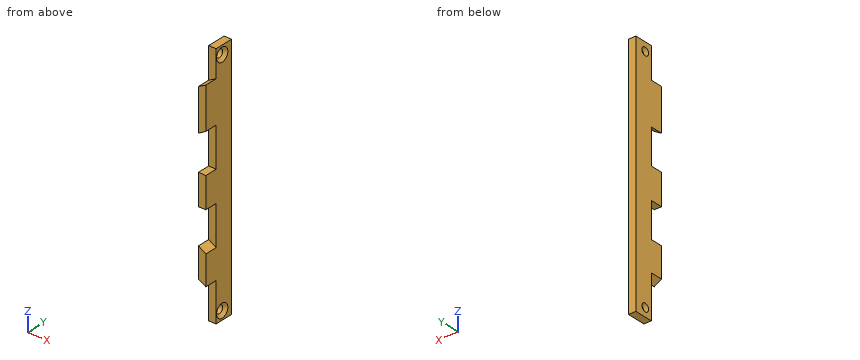
Autodesk Inventor part; units mm, degrees
ref_plane "Płaszczyzna konstrukcyjna1" through (-44.8489, 12.5303, -7) normal (0, 1, 0) x (0, 0, 1)
ref_plane "YZ Plane" through (0, 0, 0) normal (1, 0, 0) x (0, 1, 0)
ref_plane "XZ Plane" through (0, 0, 0) normal (0, 1, 0) x (-1, 0, 0)
sketch "Szkic1" plane through (0, 0, 0) normal (1, 0, 0) x (0, 1, 0)
  line L0 (0, 0) -> (10.93, 0)
  line L1 (10.93, 0) -> (10.93, -100)
  line L2 (10.93, -100) -> (0, -100)
  line L3 (0, -100) -> (0, 0)
  dimension "d0" = 10.93
  dimension "d1" = 100
extrude "Wyciągnięcie proste1" add sketch "Szkic1" along normal blind 3
sketch "Szkic2" plane through (0, 0, -100) normal (0, -1, 0) x (1, 0, 0)
  line L0 (-5, 84) -> (-8.1113, 87.1113)
  line L1 (-5, 84) -> (-4.2222, 84.7778)
  line L2 (-8.1113, 87.1113) -> (-7.3335, 87.8891)
  line L3 (-2, 60) -> (-3.1388, 64.2501)
  line L4 (-2, 60) -> (-0.9375, 60.2847)
  line L5 (-3.1388, 64.2501) -> (-2.0763, 64.5348)
  line L6 (-3.1388, 35.7499) -> (-2, 40)
  line L7 (-3.1388, 35.7499) -> (-2.0763, 35.4652)
  line L8 (-2, 40) -> (-0.9375, 39.7153)
  line L9 (-8.1113, 12.8887) -> (-5, 16)
  line L10 (-8.1113, 12.8887) -> (-7.3335, 12.1109)
  line L11 (-5, 16) -> (-4.2222, 15.2222)
  line L12 (-30.0489, 4.1) -> (-25.6489, 4.1)
  line L13 (-30.0489, 4.1) -> (-30.0489, 3)
  line L14 (-25.6489, 4.1) -> (-25.6489, 3)
  line L15 (-1.7913, 81.5519) -> (-5, 78.3431)
  line L16 (-5, 78.3431) -> (-13.7681, 87.1113)
  line L17 (-13.7681, 87.1113) -> (-10.5594, 90.32)
  line L18 (-10.5594, 90.32) -> (185.0217, 443.1577)
  arc A0 (351.0464, 277.133) -> (185.0217, 443.1577) centre (-11.203, 80.9083) ccw
  line L19 (351.0464, 277.133) -> (-1.7913, 81.5519)
  arc A1 (402.9118, 49.2349) -> (342.1425, 276.0288) centre (-8.9178, 60.424) ccw
  line L20 (402.9118, 49.2349) -> (-0.4452, 56.2755)
  line L21 (-0.4452, 56.2755) -> (-4.8284, 55.101)
  line L22 (-4.8284, 55.101) -> (-8.0378, 67.0785)
  line L23 (-8.0378, 67.0785) -> (-3.6546, 68.253)
  line L24 (-3.6546, 68.253) -> (342.1425, 276.0288)
  arc A2 (342.1425, -176.0288) -> (402.9118, 50.7651) centre (-8.9178, 39.576) ccw
  line L25 (342.1425, -176.0288) -> (-3.6546, 31.747)
  line L26 (-3.6546, 31.747) -> (-8.0378, 32.9215)
  line L27 (-8.0378, 32.9215) -> (-4.8284, 44.899)
  line L28 (-4.8284, 44.899) -> (-0.4452, 43.7245)
  line L29 (-0.4452, 43.7245) -> (402.9118, 50.7651)
  arc A3 (185.0217, -343.1577) -> (351.0464, -177.133) centre (-11.203, 19.0917) ccw
  line L30 (185.0217, -343.1577) -> (-10.5594, 9.68)
  line L31 (-10.5594, 9.68) -> (-13.7681, 12.8887)
  line L32 (-13.7681, 12.8887) -> (-5, 21.6569)
  line L33 (-5, 21.6569) -> (-1.7913, 18.4481)
  line L34 (-1.7913, 18.4481) -> (351.0464, -177.133)
  line L35 (-25.6489, 3) -> (-30.0489, 3)
  line L36 (-0.9375, 39.7153) -> (-2.0763, 35.4652)
  line L37 (-7.3335, 87.8891) -> (-4.2222, 84.7778)
  line L38 (-4.2222, 15.2222) -> (-7.3335, 12.1109)
  line L39 (-2.0763, 64.5348) -> (-0.9375, 60.2847)
  point P0 (0, 100)
  point P1 (259.8393, 226.5761)
  point P2 (359.0779, 50)
  point P3 (259.8393, -126.5761)
  point P4 (343.886, -173.1639)
  point P5 (402.9318, 50)
  point P6 (343.886, 273.1639)
extrude "Wyciągnięcie proste2" cut sketch "Szkic2" against normal blind 5 contours L0 L2 L37 L1 | L3 L5 L39 L4 | L6 L8 L36 L7 | L9 L11 L38 L10 | L15 L16 L17 L18 A0 L19 A1 L24 | L24 A1 L19 | L19 A1 A2 L29 L20 L21 L22 L23 L24 | A2 L34 L25 L26 L27 L28 L29 L20 A1 | A1 L20 L29 A2 | L34 A3 L30 L31 L32 L33 L25 A2 | A2 L25 L34
sketch "Szkic3" plane through (3, 0, 0) normal (1, 0, 0) x (0, 0, -1)
  circle A0 centre (3.5, 7.9652) radius 2
  circle A1 centre (96.5, 7.9652) radius 2
  point P0 (0, 0)
hole "Otwór1" at (3, 7.9652, -3.5) at (3, 7.9652, -96.5) direction (-1, 0, 0) diameter 3.2 depth 5 tip angle 118 countersink diameter 5.5 countersink angle 90
sketch "Szkic4" plane through (0, 5, -100) normal (0, -1, 0) x (1, 0, 0)
  line L0 (3, 100) -> (3, 84.2077)
  line L1 (0, 100) -> (3, 100)
  line L2 (0, 82.5448) -> (0, 100)
  line L3 (3, 84.2077) -> (0, 82.5448)
extrude "Wyciągnięcie proste3" add sketch "Szkic4" along normal up to surface (5 mm away)
sketch "Szkic5" plane through (0, 0, 0) normal (0, -1, 0) x (1, 0, 0)
  line L0 (4.8201, -9.9008) -> (54.794, 17.8002)
  line L1 (4.8201, -9.9008) -> (-21.7144, -24.6091)
  line L2 (-21.7144, -24.6091) -> (-5.6558, 14.396)
  line L3 (-5.6558, 14.396) -> (27.8601, 2.8705)
  line L4 (3, 0) -> (3, -27.7486)
  line L5 (0, 0) -> (0, -29.5511)
  line L6 (3, 0) -> (0, 0)
  point P0 (0, -12.5726)
  point P1 (3, -10.9097)
extrude "Wyciągnięcie proste4" cut sketch "Szkic5" against normal up to surface (5 mm away) contours L1 L5 L6 L4
sketch "Szkic6" plane through (0, 10.93, 0) normal (0, 1, 0) x (1, 0, 0)
  line L0 (0, 100) -> (0, 0)
  line L1 (0, 0) -> (3, 0)
  line L2 (3, 100) -> (3, 0)
  line L3 (0, 100) -> (3, 100)
  point P0 (0, 0)
ref_plane "Płaszczyzna konstrukcyjna1" through (-44.8489, 12.5303, -7) normal (0, 1, 0) x (0, 0, 1)
extrude "Wyciągnięcie proste5" add sketch "Szkic6" along normal up to surface (1.6003 mm away)
properties part number "przod" material "Stal, odlew"
Part model, mm, in its own coordinate system. Round coordinates to 2 decimals unless told otherwise and drop trailing zeros. Order: outer loops, then holes, each group sorted by start corner. A loop starts at its lowest first (then second) coordinate and runs counter-clockwise, first axis right, second up. Notation, with made-up numbers: M 81.25,-38 L 127.25,-38 A29 ccw 127.25,-5 Z; hole C -29,-35.75 d2. An arc over 180 degrees is marked long. Put each result on its own line as item: value. Start each with the question number.
1. Drop flat-ended pins along their axis: pin 1 (3 mm diameter, centred on y = 7.97, z = -96.5, fed in from -X); pin 2 (0.9 mm diameter, centred on x = 1, z = -67.5, fed in from -Y); pin 3 (4 mm diameter, centred on y = 7.97, z = -3.5, fed in from +X). Give the stop position or say it passes through.
2. Slice it at C-C on x = 0.6. List the corners of the cut face in (y, z).
3. Slice it at B-B on z = -96.5. List the corners of the cut face in (x, y).
4. Slice it at A-A on y = 3. List the corners of the cut face in (x, z), then the cut area to 3 significant figures.
5. Drill centre lines: probe 1 along Y at (x, z) = (0.5, -3.5); probe 2 along Z at (x, y) = (0.65, 2); probe 3 along Z at (x, y) = (0.3, 1.5). Where is each one in solid material? Low to high. Write a range as [from, to].
Findings:
1. pin 1: through
1. pin 2: y = 5
1. pin 3: x = 2.25
2. outline: M 0,-82.88 L 5,-82.88 L 5,-100 L 12.53,-100 L 12.53,0 L 5,0 L 5,-12.24 L 0,-12.24 L 0,-29.19 L 5,-29.19 L 5,-43.74 L 0,-43.74 L 0,-56.26 L 5,-56.26 L 5,-70.81 L 0,-70.81 Z; hole C 7.97,-96.5 d3.2; hole C 7.97,-3.5 d3.2
3. outline: M 0,5 L 3,5 L 3,5.22 L 1.85,6.37 L 0,6.37 Z; M 0,9.57 L 1.85,9.57 L 3,10.72 L 3,12.53 L 0,12.53 Z
4. outline: M 0,-82.54 L 3,-84.21 L 3,-72.25 L 0,-70.45 Z; M 0,-56.27 L 3,-56.22 L 3,-43.78 L 0,-43.73 Z; M 0,-29.55 L 3,-27.75 L 3,-10.91 L 0,-12.57 Z
4. area: 124 mm2
5. probe 1: [5, 6.37], [9.57, 12.53]
5. probe 2: [-82.91, -70.84], [-56.26, -43.74], [-29.16, -12.21]
5. probe 3: [-82.71, -70.63], [-56.26, -43.74], [-29.37, -12.41]
